Part model, mm, in its own coordinate system. A direction names the side the tool comes from. Round coordinates to 2 decimals unless told otherwise and drop trailing zeros. Loops run counter-clockwise (first coordinate to the right, second up) from the corner with the lowest first, then second, coordinate; pieces in that order, holes last.
from build123d import *

# Parameters (mm, degrees)
SKETCH_1_W          = 50
SKETCH_1_H          = 40
SKETCH_1_R          = 1.65
EXTRUDE_1_DEPTH     = 6
SKETCH_4_W          = 9
SKETCH_4_H          = 4
EXTRUDE_2_DEPTH     = 27
SKETCH_5_R          = 1.35
CUT_EXTRUDE_1_DEPTH = 10
EXTRUDE_3_DEPTH     = 4.05
SKETCH_8_W          = 15
SKETCH_8_H          = 27
SKETCH_8_R          = 1.5
EXTRUDE_5_DEPTH     = 8


with BuildPart() as part:
    # 草图1 → 凸台-拉伸1 (new body)
    with BuildSketch(Plane.XY):
        with Locations((234.126074566, 0)):
            Rectangle(SKETCH_1_W, SKETCH_1_H)
        with Locations((219.126074566, 0)):
            Circle(SKETCH_1_R, mode=Mode.SUBTRACT)
        with Locations((249.126074566, 0)):
            Circle(SKETCH_1_R, mode=Mode.SUBTRACT)
    extrude(amount=EXTRUDE_1_DEPTH)

    # 草图4 → 凸台-拉伸2 (add)
    with BuildSketch(Plane.XY.offset(6)):
        with Locations((217.676074566, -13.041642787)):
            Rectangle(SKETCH_4_W, SKETCH_4_H)
        with Locations((250.076074566, -13.041642787)):
            Rectangle(SKETCH_4_W, SKETCH_4_H)
    extrude(amount=EXTRUDE_2_DEPTH)

    # 草图5 → 切除-拉伸1 (cut)
    with BuildSketch(Plane.XZ.offset(15.041642787)):
        with Locations((247.876074566, 28)):
            Circle(SKETCH_5_R)
        with Locations(Location((219.876074566, 28, 0), (0, 0, 270))):
            Circle(SKETCH_5_R)
    extrude(amount=-CUT_EXTRUDE_1_DEPTH, mode=Mode.SUBTRACT)

    # 草图6 → 凸台-拉伸3 (add)
    with BuildSketch(Plane.ZY.offset(-213.176074566)):
        Polygon((6, -15.041642787), (6, -0.041642787), (33, -11.041642787), (33, -15.041642787), align=None)
    extrude(amount=EXTRUDE_3_DEPTH)

    # 草图8 → 凸台-拉伸5 (add)
    with BuildSketch(Plane(origin=(0, 20, 0), x_dir=(1, 0, 0), z_dir=(0, 1, 0))):
        with Locations((238.951074566, -19.5)):
            Rectangle(SKETCH_8_W, SKETCH_8_H)
        with Locations(Location((238.951074566, -28, 0), (0, 0, 270))):
            Circle(SKETCH_8_R, mode=Mode.SUBTRACT)
    extrude(amount=-EXTRUDE_5_DEPTH)


solid = part.part
1) Slice it at D-D, the plane x = 225.5. Give the cut face in (y, z), then the cut area to 3 significant figures.
Values:
outline: (-20, 0) - (20, 0) - (20, 6) - (-20, 6) - close
area: 240 mm2
2) Drop flat-ended pins along their axis: pin 1 Ø3.5 at (y, z) = (-6.5, 17.5) entering from +X; pin 2 Ø10 at (x, y) = (254, -12) entering from -Z; pin 3 Ø1.8 at (x, z) = (238.95, 28) entering from +Y; pin 4 Ø3 at (x, z) = (232.5, 25.5) entering from -Y. Give the stop position or say it passes through.
Values:
pin 1: stops at x = 213.18
pin 2: stops at z = 0
pin 3: passes through
pin 4: stops at y = 12
3) Slice it at C-C, the plane y = 7.5. Give the cut face in (x, z).
Values:
outline: (209.13, 0) - (259.13, 0) - (259.13, 6) - (209.13, 6) - close
4) Wall check: line 1 along Z through (x, y) = (220.5, 14.5); line 2 along Y through (x, z) = (245.5, 18); line 3 along X through (y, z) = (16.5, 12.5). Give the ranges that are in metal, low to high.
Values:
line 1: z = 0 to 6
line 2: y = 12 to 20
line 3: x = 231.45 to 246.45
5) Tool access for faces 1 (the face through (209.126, -4, 9)), 2 (the face through (245.576, -13, 19)), 3 (the face through (218, -11.042, 19)), 4 (the face through (234, 0, 6)): list every direction of +Z, -Z, +X, -X, +Y, -Y with a clear straight run to the whole face (end or side of a thin tool).
Values:
face 1: +Z, -Z, -X, +Y, -Y
face 2: +Z, -Y
face 3: +Z, +X, +Y
face 4: +Z
6) Mould opens along Y. For faces 5 (the face through (239, 20, 13)), 6 (the face through (216, -15.042, 20)), 7 (the face through (249.12, -13.07, 27.48)), 8 (the face through (247.478, 0.073, 2.958)) say: released by +Y, released by -Y, zero draft, split by the parting line, or undercut.
Values:
face 5: released by +Y
face 6: released by -Y
face 7: zero draft
face 8: undercut
7) Slice it at B-B, the plane z = 28. Give the cut face in (x, y), then the cut area to 3 significant figures.
Values:
outline: (209.13, -15.04) - (218.53, -15.04) - (218.53, -11.04) - (213.18, -11.04) - (213.18, -9) - (209.13, -9) - close; (221.23, -15.04) - (222.18, -15.04) - (222.18, -11.04) - (221.23, -11.04) - close; (231.45, 12) - (237.45, 12) - (237.45, 20) - (231.45, 20) - close; (240.45, 12) - (246.45, 12) - (246.45, 20) - (240.45, 20) - close; (245.58, -15.04) - (246.53, -15.04) - (246.53, -11.04) - (245.58, -11.04) - close; (249.23, -15.04) - (254.58, -15.04) - (254.58, -11.04) - (249.23, -11.04) - close
area: 171 mm2
8) Slice it at A-A, the plane z = 12.5. Give the cut face in (x, y), then the cut area to 3 significant figures.
Values:
outline: (209.13, -15.04) - (222.18, -15.04) - (222.18, -11.04) - (213.18, -11.04) - (213.18, -2.69) - (209.13, -2.69) - close; (231.45, 12) - (246.45, 12) - (246.45, 20) - (231.45, 20) - close; (245.58, -15.04) - (254.58, -15.04) - (254.58, -11.04) - (245.58, -11.04) - close
area: 242 mm2
